Autodesk Inventor part; units mm, degrees
ref_plane "YZ Plane" through (0, 0, 0) normal (1, 0, 0) x (0, 1, 0)
ref_plane "XZ Plane" through (0, 0, 0) normal (0, 1, 0) x (-1, 0, 0)
ref_plane "XY Plane" through (0, 0, 0) normal (0, 0, 1) x (1, 0, 0)
sketch "Sketch1" plane through (0, 0, 0) normal (0, 0, 1) x (1, 0, 0)
  circle A0 centre (0, 0) radius 7.1437
  circle A1 centre (0, 0) radius 7.9566
  circle A2 centre (0, 0) radius 9.525
  circle A3 centre (0, 0) radius 8.7122
  dimension "d0" = 14.2875
  dimension "d1" = 0.8128
  dimension "d2" = 19.05
  dimension "d3" = 0.8128
extrude "Extrusion1" add sketch "Sketch1" along normal mid plane 3.175
fillet "Fillet1" radius 0.127 2 edges at (-9.525, 0, 1.5875) (-9.525, 0, -1.5875)
chamfer "Chamfer1" distance 0.127 angle 45 2 edges at (-7.1437, 0, 1.5875) (-7.1437, 0, -1.5875)
extrude "Extrusion2" add sketch "Sketch1" along normal mid plane 2.921 contours A3
properties part number "Front Hub Bearing"
Could you check a few things on this model? Use its own coordinates, in mm. A direction names the side the tool comes from. Round coordinates to 2 decimals unless told otherwise and drop trailing zeros. Loops run counter-clockwise (first coordinate to the right, second up) from the corner with the lowest first, then second, coordinate; pieces in that order, holes last. Notation, with made-up numbers: M 38.5,87.5 L 89.5,87.5 A26 cw 89.5,120.5 Z; hole C -15,-31 d1. An arc over 180 degrees is marked long. Answer as CSV lines item,"result".
1) If I drill on probe 1 along Y at (x, z) = (0, 1.5); probe 2 along Y at (x, z) = (0, -0.75) (3 decimals); probe 3 along Y at (x, z) = (4.5, -0.2), over which ranges is the centre line in solid material (lowest first)?
From the geometry:
probe 1,"-9.52 to -8.71, -7.96 to -7.18, 7.18 to 7.96, 8.71 to 9.52"
probe 2,"-9.525 to -7.144, 7.144 to 9.525"
probe 3,"-8.39 to -5.55, 5.55 to 8.39"
2) Imagine slicing it at C-C on z = 0.25. List the corners of the cut face in (x, y) for me (3 decimals).
From the geometry:
outline,"C 0,0 d19.05; hole C 0,0 d14.287"
3) We'd pull the mould along Y, two halves only. Please class faces 1 (the cylindrical face through (-7.559, -5.796, 0.02)), 2 (the flat face through (8, -3, -1.46)), 3 (the flat face through (6, -7, -1.588)): released by +Y, released by -Y, zero draft, split by the parting line, or undercut.
From the geometry:
face 1,"split by the parting line"
face 2,"undercut"
face 3,"zero draft"
4) Which directions (+Z, -Z, +X, -X, +Y, -Y) give clear straight access to the entire face, cutting with the end or side of a thin tool? Please do faces 4 (the flat face through (8, -3, 1.46)), 5 (the cylindrical face through (6.814, -2.146, -0.02)).
From the geometry:
face 4,"+Z"
face 5,"+Z, -Z"
